Geometry check sheet. Reference: the model listing, model coordinates, mm. Coordinates: 2 decimals unless noted, no trailing zeros. Order: outer loops, then holes, each group sorted by start corner. A loop starts at its lowest first (then second) coordinate and runs counter-clockwise, first axis right, second up. Notation, with made-up numbers: (-17, 58) - (-5, 58) arc R27 cw to (-5, 78) - close; hole circle Ø8 at (50.5, -19). An arc over 180 degrees is marked (long way). Use CSV: the item, a comma, the result in double quotes. Start each with the question number.
1) Thickness scan on probe 1 along Y at (x, z) = (-76.5, -107.5); probe 2 along Z at (x, y) = (-129.5, -10). Record the ranges inside material, lowest first. Write a range as [from, to].
2) Sectioned sample at A-A, the plane z = 0. Record the cut outline in (x, y).
3) Depth check by flat-ended pin: P1, Ø1.5, axis at x = -28.5, y = -0.5, coming from the -Z side; P2, Ø1.5, axis at x = -130.5, z = -89, coming from the +Y side; P3, Ø5, axis at x = 50.5, z = -109, coming from the -Y side. Enter the tip coordinate at first touch or a pass-through.
4) Sectioned sample at B-B, the plane x = 0. Record the cut outline in (y, z).
5) Sectioned sample at C-C, the plane y = -3.5. Record the cut outline in (x, z).
from build123d import *

# Parameters (mm, degrees)
SKETCH1_R           = 165
SKETCH1_R_2         = 110
BOSS_EXTRUDE1_DEPTH = 3
SKETCH4_R           = 2.5
BOSS_EXTRUDE2_DEPTH = 16.5
CIRPATTERN1_COUNT   = 6
CUT_EXTRUDE1_DEPTH  = 10
SKETCH6_R           = 2.5
CUT_EXTRUDE2_DEPTH  = 1
CIRPATTERN5_COUNT   = 6


with BuildPart() as part:
    # Sketch1 → Boss-Extrude1 (new body)
    with BuildSketch(Plane(origin=(0, 0, 0), x_dir=(1, 0, 0), z_dir=(0, 1, 0))):
        with Locations(Location((0, 0, 0), (0, 0, 270))):
            Circle(SKETCH1_R)
        with Locations(Location((0, 0, 0), (0, 0, 270))):
            Circle(SKETCH1_R_2, mode=Mode.SUBTRACT)
    extrude(amount=BOSS_EXTRUDE1_DEPTH)

    # Sketch4 → Boss-Extrude2 (add)
    with BuildSketch(Plane.XZ):
        with Locations(Location((-11.943664818, 157.046486337, 0), (0, 0, 90))):
            Circle(SKETCH4_R)
    boss_extrude2 = extrude(amount=BOSS_EXTRUDE2_DEPTH)

    # CirPattern1: Boss-Extrude2 ×6 about axis
    cirpattern1_axis = Axis((0, 0, 0), (0, 1, 0))
    for i in range(1, CIRPATTERN1_COUNT):
        add(boss_extrude2.rotate(cirpattern1_axis, i * 360 / CIRPATTERN1_COUNT))

    # Sketch5 → Cut-Extrude1 (cut)
    with BuildSketch(Plane(origin=(0, 0, 0), x_dir=(-1, 0, 0), z_dir=(0, -1, 0))):
        with BuildLine():
            Line((-139.418207286, -55.668125577), (-151.59368138, -39.414458013))
            Line((-151.59368138, -39.414458013), (-153.890000313, -41.134609577))
            Line((-153.890000313, -41.134609577), (-160.156367767, -43.657048272))
            ThreePointArc((-160.156367767, -43.657048272), (-154.417811813, -60.91912175), (-146.824907269, -77.449639157))
            Line((-146.824907269, -77.449639157), (-139.16221183, -66.09993074))
            ThreePointArc((-139.16221183, -66.09993074), (-137.624058072, -60.843140968), (-139.418207286, -55.668125577))
        make_face()
    extrude(amount=-CUT_EXTRUDE1_DEPTH, mode=Mode.SUBTRACT)

    # Sketch6 → Cut-Extrude2 (cut)
    with BuildSketch(Plane(origin=(0, 3, 0), x_dir=(1, 0, 0), z_dir=(0, 1, 0))):
        with Locations(Location((11.943664818, 157.046486337, 0), (0, 0, 270))):
            Circle(SKETCH6_R)
    cut_extrude2 = extrude(amount=-CUT_EXTRUDE2_DEPTH, mode=Mode.SUBTRACT)

    # CirPattern5: Cut-Extrude2 ×6 about axis
    cirpattern5_axis = Axis((0, 0, 0), (0, 1, 0))
    for i in range(1, CIRPATTERN5_COUNT):
        add(cut_extrude2.rotate(cirpattern5_axis, i * 360 / CIRPATTERN5_COUNT), mode=Mode.SUBTRACT)


solid = part.part
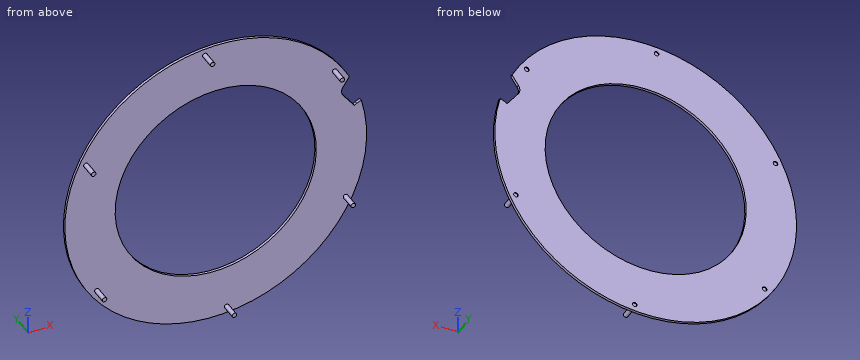
Evaluation:
1,probe 1,"[0, 3]"
1,probe 2,"[-91.31, -86.42]"
2,outline,"(-165, 0) - (-110, 0) - (-110, 3) - (-165, 3) - close; (110, 0) - (165, 0) - (165, 3) - (110, 3) - close"
3,P1,"z = -162.62"
3,P2,"y = 2"
3,P3,"y = 0"
4,outline,"(0, -165) - (3, -165) - (3, -110) - (0, -110) - close; (0, 110) - (3, 110) - (3, 165) - (0, 165) - close"
5,outline,"circle Ø5 at (-141.98, 68.18); circle Ø5 at (-130.03, -88.87); circle Ø5 at (-11.94, 157.05); circle Ø5 at (11.94, -157.05); circle Ø5 at (130.03, 88.87); circle Ø5 at (141.98, -68.18)"
